```python
from build123d import *

# Parameters (mm, degrees)
SKETCH1_R            = 6.235
BOSS_EXTRUDE1_DEPTH  = 1.05
SKETCH2_W            = 5.87
SKETCH2_H            = 0.86
SKETCH2_W_2          = 0.86
SKETCH2_H_2          = 5.87
BOSS_EXTRUDE5_DEPTH  = 11.52
SKETCH10_W           = 0.86
SKETCH10_H           = 7.57
BOSS_EXTRUDE6_DEPTH  = 60.27
SKETCH11_W           = 7.57
SKETCH11_H           = 0.86
BOSS_EXTRUDE8_DEPTH  = 60.27
SKETCH15_R           = 4.13
BOSS_EXTRUDE9_DEPTH  = 0.76
SKETCH16_W           = 1.010303068
SKETCH16_H           = 7.6
SKETCH16_W_2         = 7.6
SKETCH16_H_2         = 1.157256242
BOSS_EXTRUDE10_DEPTH = 2.71
SKETCH17_R           = 3.99
BOSS_EXTRUDE11_DEPTH = 1.25
SKETCH18_W           = 2.18
SKETCH18_H           = 0.9
SKETCH18_W_2         = 0.9
SKETCH18_H_2         = 2.18
BOSS_EXTRUDE13_DEPTH = 0.5
SKETCH19_R           = 4.36
BOSS_EXTRUDE14_DEPTH = 3.46


with BuildPart() as part:
    # Sketch1 → Boss-Extrude1 (new body)
    with BuildSketch(Plane(origin=(0, 0, 0), x_dir=(0, 0, -1), z_dir=(1, 0, 0))):
        Circle(SKETCH1_R)
    extrude(amount=BOSS_EXTRUDE1_DEPTH)

    # Sketch2 → Boss-Extrude5 (add)
    with BuildSketch(Plane(origin=(1.05, 0, 0), x_dir=(0, 0, -1), z_dir=(1, 0, 0))):
        Rectangle(SKETCH2_W, SKETCH2_H)
        Rectangle(SKETCH2_W_2, SKETCH2_H_2)
    extrude(amount=BOSS_EXTRUDE5_DEPTH)

    # Sketch10 → Boss-Extrude6 (add)
    with BuildSketch(Plane(origin=(12.57, 0, 0), x_dir=(0, 0, -1), z_dir=(1, 0, 0))):
        Rectangle(SKETCH10_W, SKETCH10_H)
    extrude(amount=BOSS_EXTRUDE6_DEPTH)

    # Sketch11 → Boss-Extrude8 (add)
    with BuildSketch(Plane(origin=(12.57, 0, 0), x_dir=(0, 0, -1), z_dir=(1, 0, 0))):
        Rectangle(SKETCH11_W, SKETCH11_H)
    extrude(amount=BOSS_EXTRUDE8_DEPTH)

    # Sketch15 → Boss-Extrude9 (add)
    with BuildSketch(Plane(origin=(72.84, 0, 0), x_dir=(0, 0, -1), z_dir=(1, 0, 0))):
        Circle(SKETCH15_R)
    extrude(amount=BOSS_EXTRUDE9_DEPTH)

    # Sketch16 → Boss-Extrude10 (add)
    with BuildSketch(Plane(origin=(73.6, 0, 0), x_dir=(0, 0, -1), z_dir=(1, 0, 0))):
        with Locations((-0.018369147, 0)):
            Rectangle(SKETCH16_W, SKETCH16_H)
        with Locations((0, 0.045922867)):
            Rectangle(SKETCH16_W_2, SKETCH16_H_2)
    extrude(amount=BOSS_EXTRUDE10_DEPTH)

    # Sketch17 → Boss-Extrude11 (add)
    with BuildSketch(Plane(origin=(76.31, 0, 0), x_dir=(0, 0, -1), z_dir=(1, 0, 0))):
        Circle(SKETCH17_R)
    extrude(amount=BOSS_EXTRUDE11_DEPTH)

    # Sketch18 → Boss-Extrude13 (add)
    with BuildSketch(Plane(origin=(77.56, 0, 0), x_dir=(0, 0, -1), z_dir=(1, 0, 0))):
        with Locations((1.54, 0)):
            Rectangle(SKETCH18_W, SKETCH18_H)
        with Locations((0, 1.54)):
            Rectangle(SKETCH18_W_2, SKETCH18_H_2)
        with Locations((-1.54, 0)):
            Rectangle(SKETCH18_W, SKETCH18_H)
        Rectangle(SKETCH18_W_2, SKETCH18_H)
        with Locations((0, -1.54)):
            Rectangle(SKETCH18_W_2, SKETCH18_H_2)
    extrude(amount=BOSS_EXTRUDE13_DEPTH)

    # Sketch19 → Boss-Extrude14 (add)
    with BuildSketch(Plane(origin=(78.06, 0, 0), x_dir=(0, 0, -1), z_dir=(1, 0, 0))):
        Circle(SKETCH19_R)
    extrude(amount=BOSS_EXTRUDE14_DEPTH)

    # Boss-Extrude15 cone 1 section (through the dimple's axis) → Boss-Extrude15 (revolve)
    with BuildSketch(Plane(origin=(81.52, 0, 0), x_dir=(0, 0, 1), z_dir=(0, 1, 0))):
        Polygon((0, 0), (4.36, 0), (0, 3.052904867), align=None)
    revolve(axis=Axis((81.52, 0, 0), (1, 0, 0)))


solid = part.part
```
Read the model definition and answer for the solid it produces. Units are mm, in the model's axes. A direction names the side the tool comes from. Give positions to 0.01 mm unless a question says otherwise; leave off trailing zeros. Write each loop counter-clockwise with the first axis right and the second up, starting at its lowest first coordinate (ties: lowest second). Pieces come first, ordered by that corner, then holes. Notation, with made-up numbers: M 53,42 L 79,42 A18 ccw 79,60 Z; hole C 59.5,-31.5 d7. An arc over 180 degrees is marked long. Put each result on its own line as item: value. Start each with the question number.
1. Consider line 1 along Y through (x, z) = (30.5, 2.75); line 2 along X through (y, z) = (-1.5, 1.5); line 3 along X through (y, z) = (-5, -0.5). Determine where each line is inside the solid, lowest interval first.
2. The part is cut by section A-A, the plane x = 70. Give the vertices of the cut face in (y, z) (3 decimals), and give its area (3 significant figures).
3. For a pull along X with two mould halves and no side action, classify faces 5 (the flat face through (0, 0, 0)), 6 (the flat face through (77.56, -1, -1)), 7 (the cylindrical face through (76.926, -2.428, 3.166)) as released by +X, released by -X, zero draft, split by the parting line, or undercut.
4. Which of the six approach directions +Z, -Z, +X, -X, +Y, -Y give full straight-line access (tool end or side, diameter ignored) to faces 1 (the flat face through (36, -2, -0.43)), 2 (the flat face through (36, 2, -0.43)), 3 (the flat face through (36, -0.43, 2)), 4 (the flat face through (73.6, -1, -1))?
5. Each of these flat-tipped pins is pushed along its axis until it touches: pin 1 Ø1.5 at (x, z) = (15.5, 4.5) entering from +Y; pin 2 Ø4 at (y, z) = (-2, -0.5) entering from +X; pin 3 Ø0.7 at (x, z) = (6.5, 0) entering from +Y (3 decimals); pin 4 Ø0.9 at (y, z) = (-3.5, 0) entering from -X. Where does it stop, or does it pass through?
Final values:
1. line 1: y = -0.43 to 0.43
1. line 2: x = 0 to 1.05, 72.84 to 73.6, 76.31 to 77.56, 78.06 to 83.09
1. line 3: x = 0 to 1.05
2. outline: M -3.785,-0.43 L -0.43,-0.43 L -0.43,-3.785 L 0.43,-3.785 L 0.43,-0.43 L 3.785,-0.43 L 3.785,0.43 L 0.43,0.43 L 0.43,3.785 L -0.43,3.785 L -0.43,0.43 L -3.785,0.43 Z
2. area: 12.3 mm²
3. face 5: released by -X
3. face 6: undercut
3. face 7: undercut
4. face 1: -Z, -Y
4. face 2: -Z, +Y
4. face 3: +Z, -Y
4. face 4: none
5. pin 1: stops at y = 0.43
5. pin 2: stops at x = 84.53
5. pin 3: stops at y = 2.935
5. pin 4: stops at x = 0
